CAD build for the part. Positions are in the model's coordinates, mm. Face numbers are marked on the shaded views. A direction names the side the tool comes from. Round coordinates to 2 decimals unless told otherwise and drop trailing zeros. Order: outer loops, then holes, each group sorted by start corner. A loop starts at its lowest first (then second) coordinate and runs counter-clockwise, first axis right, second up. Notation, with made-up numbers: (54.25, -16) - (79.25, -16) arc R30 cw to (79.25, 7) - close; hole circle Ø10 at (33, 50). An arc over 180 degrees is marked (long way). Use one line per item in the form item = value. Start each with the question number.
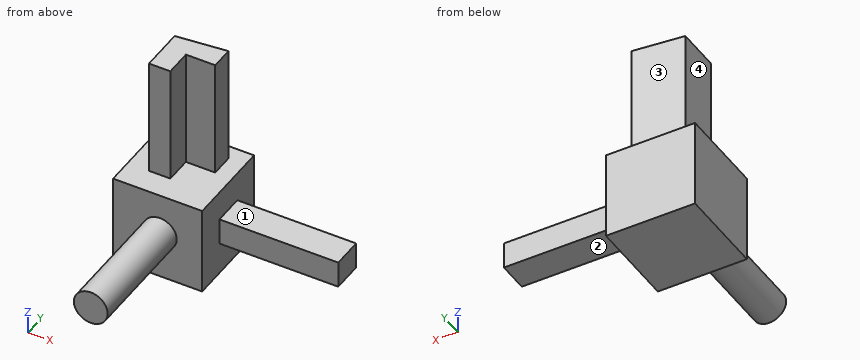
from build123d import *

# Parameters (mm, degrees)
F0_W     = 19.05
F0_H     = 19.05
F1_DEPTH = 19.05
F2_R     = 3.608041
F3_DEPTH = 25.4
F4_W     = 6.560533
F4_H     = 5.704813
F5_DEPTH = 25.4
F7_DEPTH = 25.4


with BuildPart() as f1:
    # F0 (on Top) → F1 (new body)
    with BuildSketch(Plane.XY):
        with Locations((-18.726731, 9.476246)):
            Rectangle(F0_W, F0_H)
    extrude(amount=F1_DEPTH)

    # F2 (on face) → F3 (join)
    with BuildSketch(Plane.XZ.offset(0.048754)):
        with Locations((-18.255401, 10.126043)):
            Circle(F2_R)
    extrude(amount=F3_DEPTH)

    # F4 (on face) → F5 (join)
    with BuildSketch(Plane.YZ.offset(-9.201731)):
        with Locations((9.555563, 9.840802)):
            Rectangle(F4_W, F4_H)
    extrude(amount=F5_DEPTH)

    # F6 (on face) → F7 (join)
    with BuildSketch(Plane.XY.offset(19.05)):
        Polygon((-12.835828, 15.830856), (-23.674972, 14.689893), (-23.674972, 5.276952), (-19.111123, 5.276952), (-19.111123, 10.981766), (-12.835828, 10.981766), align=None)
    extrude(amount=F7_DEPTH)


solid = f1.part
(1) Slice it at B-B (x = -6.5). Give the cut face in (y, z).
(2) Slice it at C-C (y = 16.5). Give the cut face in (x, z), and give its area (3 significant figures).
(3) Flat gauge pins, fed straight in: P1, Ø2, axis at x = 4.5, y = 11, coming from the -Z side; P2, Ø1.5, axis at y = 12.5, z = 34, coming from the +X side; P3, Ø2, axis at x = 7, y = 9, coming from the +Z side; P4, Ø9.5, axis at x = -15.5, y = 10, coming from the +Z side. Where does each tip first touch, or does it go through?
(4) Wall check: line 1 (Y direction, x = -1, z = 8); line 2 (Z direction, x = -18, y = -4.5); line 3 (Y direction, x = -12, z = 12). Give the ranges that are in metal, low to high. Write a range as [from, to].
(5) Which spindle directions (+Z, -Z, +X, -X, +Y, -Y) get a long thin tool onto all of the face, cutting with end or side? Do the marked faces 1, 2, 3 and 4. Say none if no direction does.
(6) Slice it at A-A (z = 9.5). Give the cut face in (x, y), and give its area (3 significant figures).
(7) Slice it at D-D (z = 33). Give the cut face in (x, y).
Results list:
q1.outline = (6.28, 6.99) - (12.84, 6.99) - (12.84, 12.69) - (6.28, 12.69) - close
q2.outline = (-28.25, 0) - (-9.2, 0) - (-9.2, 19.05) - (-28.25, 19.05) - close
q2.area = 363 mm²
q3.P1 = 6.99
q3.P2 = -12.84
q3.P3 = 12.69
q3.P4 = 44.45
q4.line_1 = [6.28, 12.84]
q4.line_2 = [6.53, 13.73]
q4.line_3 = [-0.05, 19]
q5.face_1 = +Z, +X, +Y, -Y
q5.face_2 = -Z, +X, +Y, -Y
q5.face_3 = +Z, -X, +Y
q5.face_4 = +Z, -X, +Y, -Y
q6.outline = (-28.25, -0.05) - (-21.81, -0.05) - (-21.81, -25.45) - (-14.7, -25.45) - (-14.7, -0.05) - (-9.2, -0.05) - (-9.2, 6.28) - (16.2, 6.28) - (16.2, 12.84) - (-9.2, 12.84) - (-9.2, 19) - (-28.25, 19) - close
q6.area = 710 mm²
q7.outline = (-23.67, 5.28) - (-19.11, 5.28) - (-19.11, 10.98) - (-12.84, 10.98) - (-12.84, 15.83) - (-23.67, 14.69) - close
